Check sheet for the modelled part. Datum: model origin and axes. Units: mm. Give positions to 0.01 mm unless a question says otherwise; leave off trailing zeros. Loops run counter-clockwise (first coordinate to the right, second up) from the corner with the lowest first, then second, coordinate; pieces in that order, holes last.
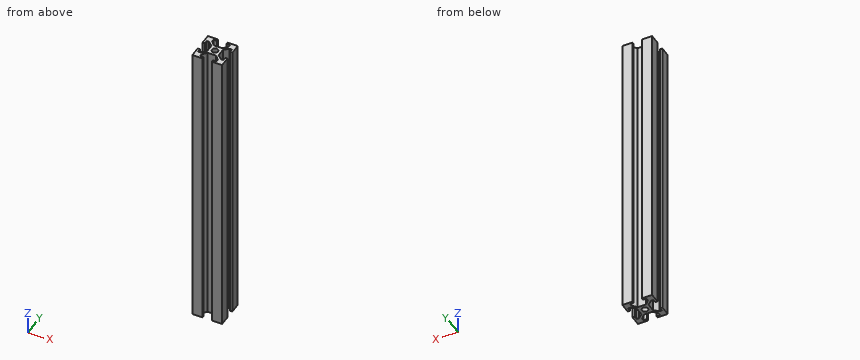
```python
from build123d import *

# Parameters (mm, degrees)
SKETCH1_R           = 2
BOSS_EXTRUDE1_DEPTH = 100


with BuildPart() as part:
    # Sketch1 → Boss-Extrude1 (new, symmetric)
    with BuildSketch(Plane.XY):
        Polygon((10, 4.610379336), (10, 10), (4.610379336, 10), (3.1, 10), (3.1, 8.5), (5.5, 8.5), (5.5, 6.860660172), (2.839339828, 3.9), (0.519615242, 3.9), (-0.519615242, 3.9), (-2.839339828, 3.9), (-5.5, 6.860660172), (-5.5, 8.5), (-3.1, 8.5), (-3.1, 10), (-4.610379336, 10), (-10, 10), (-10, 4.610379336), (-10, 3.1), (-8.5, 3.1), (-8.5, 5.5), (-6.860660172, 5.5), (-3.9, 2.839339828), (-3.9, 0.519615242), (-3.9, -0.519615242), (-3.9, -2.839339828), (-6.860660172, -5.5), (-8.5, -5.5), (-8.5, -3.1), (-10, -3.1), (-10, -4.610379336), (-10, -10), (-4.610379336, -10), (-3.1, -10), (-3.1, -8.5), (-5.5, -8.5), (-5.5, -6.860660172), (-2.839339828, -3.9), (-0.519615242, -3.9), (0.519615242, -3.9), (2.839339828, -3.9), (5.5, -6.860660172), (5.5, -8.5), (3.1, -8.5), (3.1, -10), (4.610379336, -10), (10, -10), (10, -4.610379336), (10, -3.1), (8.5, -3.1), (8.5, -5.5), (6.860660172, -5.5), (3.9, -2.839339828), (3.9, -0.519615242), (3.9, 0.519615242), (3.9, 2.839339828), (6.860660172, 5.5), (8.5, 5.5), (8.5, 3.1), (10, 3.1), align=None)
        Circle(SKETCH1_R, mode=Mode.SUBTRACT)
    extrude(amount=BOSS_EXTRUDE1_DEPTH, both=True)


solid = part.part
```
(1) Section check A-A on y = 0. Record the boundary of the cut face in (x, z), plus the area to 3 significant figures.
(2) Material ranges on line 1 (Y direction, x = 0, z = -15); line 2 (X direction, y = 3.75, z = -82); line 3 (Y direction, x = 9.25, z = -84), recorded low to high.
(3) Gauge pin test, flat ends, axial feed: pin 1 Ø1 at (x, z) = (-1.5, 72.5) entering from -Y; pin 2 Ø1.5 at (x, z) = (0, -78.5) entering from +Y; pin 3 Ø3 at (x, z) = (-1.5, 16) entering from +Y; pin 4 Ø3 at (x, y) = (-1, -8) entering from -Z. Record the tip position at first contact, or that the pin passes through.
Computed values:
1. outline: (-3.9, -100) - (-2, -100) - (-2, 100) - (-3.9, 100) - close; (2, -100) - (3.9, -100) - (3.9, 100) - (2, 100) - close
1. area: 760 mm2
2. line 1: y = -3.9 to -2, 2 to 3.9
2. line 2: x = -10 to -8.5, -4.91 to 4.91, 8.5 to 10
2. line 3: y = -10 to -3.1, 3.1 to 10
3. pin 1: stops at y = -3.9
3. pin 2: stops at y = 3.9
3. pin 3: stops at y = 4.08
3. pin 4: passes through
